Read the model definition and answer for the solid it produces. Units are mm, in the model's axes. A direction names the side the tool comes from. Coordinates: 2 decimals unless noted, no trailing zeros. Order: outer loops, then holes, each group sorted by start corner. A loop starts at its lowest first (then second) coordinate and runs counter-clockwise, first axis right, second up. Notation, with made-up numbers: (45, 46) - (97, 46) arc R29 cw to (97, 73) - close; hole circle Ø10 at (50.5, 61.25). An arc over 180 degrees is marked (long way). Use one line per item in the form item = value.
```python
from build123d import *

# Parameters (mm, degrees)
F1_DEPTH = 304.8
F2_W     = 38.1
F2_H     = 38.1
F3_DEPTH = 304.8
F4_R     = 7.9375
F5_DEPTH = 50.8


with BuildPart() as f1:
    # F0 (on Front) → F1 (new body)
    with BuildSketch(Plane.XZ):
        with BuildLine():
            Line((-44.45, 0), (-6.35, 0))
            ThreePointArc((-6.35, 0), (-1.859872, 1.859872), (0, 6.35))
            Line((0, 6.35), (0, 44.45))
            ThreePointArc((0, 44.45), (-1.859872, 48.940128), (-6.35, 50.8))
            Line((-6.35, 50.8), (-44.45, 50.8))
            ThreePointArc((-44.45, 50.8), (-48.940128, 48.940128), (-50.8, 44.45))
            Line((-50.8, 44.45), (-50.8, 6.35))
            ThreePointArc((-50.8, 6.35), (-48.940128, 1.859872), (-44.45, 0))
        make_face()
    extrude(amount=F1_DEPTH)

    # F2 (on face) → F3 (cut)
    with BuildSketch(Plane.XZ.offset(304.8)):
        with Locations((-25.4, 25.4)):
            Rectangle(F2_W, F2_H)
    extrude(amount=-F3_DEPTH, mode=Mode.SUBTRACT)

    # F4 (on face) → F5 (cut)
    with BuildSketch(Plane.YZ):
        with Locations((-203.2, 25.4)):
            Circle(F4_R)
    extrude(amount=-F5_DEPTH, mode=Mode.SUBTRACT)


solid = f1.part
```
(1) The mould has two halves that part along Y. Classify faces 3 (the flat face through (-3, 0, 26)), 4 (the cylindrical face through (-3.13, -211.13, 25.75)), 5 (the cylindrical face through (-47.58, -211.13, 25.75)), 6 (the cylindrical face through (-48.89, -150.27, 48.99)): +Y half, -Y half, draft (parallel to the pull), parting line (faces both ways), or undercut.
Answer list:
face_3 = +Y half
face_4 = undercut
face_5 = undercut
face_6 = draft
(2) Given pin 1 Ø14.5 at (y, z) = (-203.2, 25.4) entering from +X, flat-ended and moving along its own axis, determine where the tip first touches the part or whether it passes through.
Answer list:
pin_1 = through
(3) Which of the six approach directions +Z, -Z, +X, -X, +Y, -Y give full straight-line access (tool end or side, diameter ignored) to faces 1 (the flat face through (-26, -155, 44.45)), 2 (the flat face through (-50.8, -150, 26))?
Answer list:
face_1 = +Y, -Y
face_2 = +Z, -Z, -X, +Y, -Y
(4) Section C-C, the plane z = 13.5 is taken. Write down the section's boundary in (x, y), then the cut area to 3 significant figures.
Answer list:
outline = (-50.8, -304.8) - (-44.45, -304.8) - (-44.45, 0) - (-50.8, 0) - close; (-6.35, -304.8) - (0, -304.8) - (0, 0) - (-6.35, 0) - close
area = 3,870 mm2
(5) Section A-A, the plane y = -203.2 is taken. Write down the section's boundary in (x, z).
Answer list:
outline = (-50.8, 6.35) arc R6.35 ccw to (-44.45, 0) - (-6.35, 0) arc R6.35 ccw to (0, 6.35) - (0, 17.46) - (-6.35, 17.46) - (-6.35, 6.35) - (-44.45, 6.35) - (-44.45, 17.46) - (-50.8, 17.46) - close; (-50.8, 33.34) - (-44.45, 33.34) - (-44.45, 44.45) - (-6.35, 44.45) - (-6.35, 33.34) - (0, 33.34) - (0, 44.45) arc R6.35 ccw to (-6.35, 50.8) - (-44.45, 50.8) arc R6.35 ccw to (-50.8, 44.45) - close
(6) Section D-D, the plane z = 25.4 is taken. Write down the section's boundary in (x, y), then the cut area to 3 significant figures.
Answer list:
outline = (-50.8, -304.8) - (-44.45, -304.8) - (-44.45, -211.14) - (-50.8, -211.14) - close; (-50.8, -195.26) - (-44.45, -195.26) - (-44.45, 0) - (-50.8, 0) - close; (-6.35, -304.8) - (0, -304.8) - (0, -211.14) - (-6.35, -211.14) - close; (-6.35, -195.26) - (0, -195.26) - (0, 0) - (-6.35, 0) - close
area = 3,670 mm2
(7) Straight lines are drawn through the part: L1, parallel to Z at x = -21, y = -51.5; L2, parallel to Y at x = -47, z = 25; L3, parallel to X at y = -118, z = 37. For each, find the intervals that lie inside material, in ascending order.
Answer list:
L1 = 0 to 6.35, 44.45 to 50.8
L2 = -304.8 to -211.13, -195.27 to 0
L3 = -50.8 to -44.45, -6.35 to 0
(8) Section B-B, the plane x = -25 is taken. Write down the section's boundary in (y, z), then the cut area to 3 significant figures.
Answer list:
outline = (-304.8, 0) - (0, 0) - (0, 6.35) - (-304.8, 6.35) - close; (-304.8, 44.45) - (0, 44.45) - (0, 50.8) - (-304.8, 50.8) - close
area = 3,870 mm2
